Geometry: final body of the model. Coordinates: model frame, mm. Face numbers are marked on the shaded views. A direction names the side the tool comes from. Round coordinates to 2 decimals unless told otherwise and drop trailing zeros. Loops run counter-clockwise (first coordinate to the right, second up) from the corner with the lowest first, then second, coordinate; pieces in that order, holes last. Notation, with made-up numbers: M 36.5,43 L 79.5,43 A27 ccw 79.5,65 Z; hole C -22,-9.5 d8. An arc over 180 degrees is marked long. Return JSON: item names as keys, results as strings.
from build123d import *

# Parameters (mm, degrees)
SKETCH_1_W                   = 30
SKETCH_1_H                   = 37
EXTRUDE_1_DEPTH              = 8
EXTRUDE_2_DEPTH              = 8
EXTRUDE_3_DEPTH              = 3.8
HOLE_WIZARD_M6_1_D           = 6.6
HOLE_WIZARD_M6_1_CSINK_D     = 12.6
HOLE_WIZARD_M6_1_CSINK_ANGLE = 90
HOLE_WIZARD_M6_2_D           = 6.6
HOLE_WIZARD_M6_2_CSINK_D     = 12.6
HOLE_WIZARD_M6_2_CSINK_ANGLE = 90


with BuildPart() as part:
    # 草图1 → 凸台-拉伸1 (new body)
    with BuildSketch(Plane.XY):
        Rectangle(SKETCH_1_W, SKETCH_1_H)
    extrude(amount=EXTRUDE_1_DEPTH)

    # 草图2 → 凸台-拉伸2 (add)
    with BuildSketch(Plane(origin=(0, 18.5, 0), x_dir=(1, 0, 0), z_dir=(0, 1, 0))):
        with BuildLine():
            Line((-15, -8), (15, -8))
            Line((15, -8), (15, 12))
            ThreePointArc((15, 12), (0, 27), (-15, 12))
            Line((-15, 12), (-15, -8))
        make_face()
    extrude(amount=-EXTRUDE_2_DEPTH)

    # 草图5 → 凸台-拉伸3 (add)
    with BuildSketch(Plane(origin=(15, 0, 0), x_dir=(0, 0, -1), z_dir=(1, 0, 0))):
        Polygon((12, 10.5), (0, 10.5), (0, 0), align=None)
    extrude_3 = extrude(amount=-EXTRUDE_3_DEPTH)

    # 镜向1: 凸台-拉伸3 across plane
    add(extrude_3.mirror(Plane(origin=(0, 0, 0), x_dir=(0, 0, 1), z_dir=(1, 0, 0))))

    # M6 平锥沉头螺钉的锥形沉头孔1 (through all)
    with Locations(Plane(origin=(0, 0, 0), x_dir=(-1, 0, 0), z_dir=(0, 0, -1))):
        with Locations((0, -1.5)):
            CounterSinkHole(HOLE_WIZARD_M6_1_D / 2, HOLE_WIZARD_M6_1_CSINK_D / 2, counter_sink_angle=HOLE_WIZARD_M6_1_CSINK_ANGLE)

    # M6 平锥沉头螺钉的锥形沉头孔2 (through all)
    with Locations(Plane.XZ.offset(-10.5)):
        with Locations((0, -12)):
            CounterSinkHole(HOLE_WIZARD_M6_2_D / 2, HOLE_WIZARD_M6_2_CSINK_D / 2, counter_sink_angle=HOLE_WIZARD_M6_2_CSINK_ANGLE)


solid = part.part
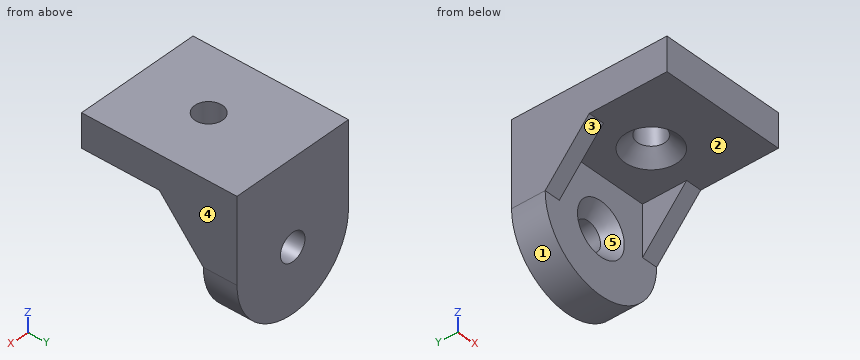
Q1. Material intervals for L1, parallel to Y at x = 0, z = 4.95; L2, parallel to X at y = -1.5, z = 5.65; L3, parallel to Y at x = -0.25, z = -20, sorted ascending.
Determined:
{"L1": "y = -18.5 to -4.8, 1.8 to 18.5", "L2": "x = -15 to -3.3, 3.3 to 15", "L3": "y = 10.5 to 18.5"}
Q2. Pin query (flat end, axial travel): pin 1 (1.5 mm diameter, centred on x = 6.5, z = -5.5, fed in from -Y); pin 2 (6 mm diameter, centred on x = 11, y = -8, fed in from -Z); pin 3 (7.5 mm diameter, centred on x = 0, y = -1.5, fed in from -Z). Return the tip coordinate at first contact, or that it passes through.
Determined:
{"pin 1": "stops at y = 10.5", "pin 2": "stops at z = 0", "pin 3": "stops at z = 2.55"}
Q3. Section query A-A (y = -1.5). Output: boundary loops of the cut face in (x, z), plus the area to 3 significant figures.
Determined:
{"outline": "M -15,0 L -6.3,0 L -3.3,3 L -3.3,8 L -15,8 Z; M 3.3,3 L 6.3,0 L 15,0 L 15,8 L 3.3,8 Z", "area": "178 mm^2"}
Q4. Reachability of the marked faces 1 and 2 from +Z, -Z, +X, -X, +Y, -Y: full face, straight path, thin tool, end or side. Return the list, or none.
Determined:
{"face 1": "-Z, +Y, -Y", "face 2": "-Z, -Y"}
Q5. Section query D-D (z = -2). Output: boundary loops of the cut face in (x, y).
Determined:
{"outline": "M -15,1.75 L -11.2,1.75 L -11.2,10.5 L 11.2,10.5 L 11.2,1.75 L 15,1.75 L 15,18.5 L -15,18.5 Z"}
Q6. Section query B-B (x = 0). Output: boundary loops of the cut face in (y, z), plus the area to 3 significant figures.
Determined:
{"outline": "M -18.5,0 L -7.8,0 L -4.8,3 L -4.8,8 L -18.5,8 Z; M 1.8,3 L 4.8,0 L 10.5,0 L 10.5,-5.7 L 13.5,-8.7 L 18.5,-8.7 L 18.5,8 L 1.8,8 Z; M 10.5,-27 L 18.5,-27 L 18.5,-15.3 L 13.5,-15.3 L 10.5,-18.3 Z", "area": "388 mm^2"}
Q7. Pull-direction query (Z, two-part tool) for the marked faces 3, 4 and 5; classes: pulls with the +Z half, pulls with the -Z half, needs draft (parallel to the pull), parting line crosses it, or undercut.
Determined:
{"face 3": "pulls with the -Z half", "face 4": "needs draft", "face 5": "undercut"}
Q8. Section query C-C (z = 4). Output: boundary loops of the cut face in (x, y).
Determined:
{"outline": "M -15,-18.5 L 15,-18.5 L 15,18.5 L -15,18.5 Z; hole C 0,-1.5 d6.6"}
